from build123d import *

# Parameters (mm, degrees)
SKETCH_1_R             = 28.9
EXTRUDE_1_DEPTH        = 1.6
CHAMFER_1_SIZE         = 0.8
SKETCH_2_R             = 23.75
EXTRUDE_2_DEPTH        = 20
HOLE_WIZARD_M4_1_D     = 3.3
HOLE_WIZARD_M4_1_DEPTH = 9.008579979
HOLE_WIZARD_M4_1_TIP   = 0.991420021
SKETCH_3_R             = 7.5
CUT_EXTRUDE_1_DEPTH    = 4
SKETCH_7_R             = 3.9
EXTRUDE_3_DEPTH        = 3.5
SKETCH_8_R             = 2.34
CUT_EXTRUDE_2_DEPTH    = 10
SKETCH_9_R             = 2
CUT_EXTRUDE_3_DEPTH    = 10


with BuildPart() as part:
    # 草图1 → 凸台-拉伸1 (new body)
    with BuildSketch(Plane(origin=(0, 0, 0), x_dir=(1, 0, 0), z_dir=(0, 1, 0))):
        with Locations(Location((0, 0, 0), (0, 0, 270))):
            Circle(SKETCH_1_R)
    extrude(amount=EXTRUDE_1_DEPTH)

    # 倒角1
    chamfer_1_edges = [part.edges().sort_by_distance(p)[0] for p in [
        (0, 1.6, -28.9),
    ]]
    chamfer(chamfer_1_edges, length=CHAMFER_1_SIZE)

    # 草图2 → 凸台-拉伸2 (add)
    with BuildSketch(Plane.XZ):
        with Locations(Location((0, 0, 0), (0, 0, 270))):
            Circle(SKETCH_2_R)
    extrude(amount=EXTRUDE_2_DEPTH)

    # M4 螺纹孔的螺纹孔钻头1
    with Locations(Plane(origin=(0, 1.6, 0), x_dir=(1, 0, 0), z_dir=(0, 1, 0))):
        with Locations((-17.25, 0), (-8.625, 14.938938215), (8.625, 14.938938215), (17.25, 0), (8.625, -14.938938215), (-8.625, -14.938938215)):
            Hole(HOLE_WIZARD_M4_1_D / 2, depth=HOLE_WIZARD_M4_1_DEPTH)
            with Locations((0, 0, -(HOLE_WIZARD_M4_1_DEPTH + HOLE_WIZARD_M4_1_TIP / 2))):  # 118° drill point
                Cone(0, HOLE_WIZARD_M4_1_D / 2, HOLE_WIZARD_M4_1_TIP, mode=Mode.SUBTRACT)

    # 草图3 → 切除-拉伸1 (cut)
    with BuildSketch(Plane(origin=(0, 1.6, 0), x_dir=(1, 0, 0), z_dir=(0, 1, 0))):
        with Locations(Location((0, 0, 0), (0, 0, 270))):
            Circle(SKETCH_3_R)
        with BuildLine():
            Line((-2.628287969, 9.808904238), (-4.34330439, 16.209432654))
            ThreePointArc((-4.34330439, 16.209432654), (-4.081182154, 17.827981129), (-2.696831759, 18.706605744))
            ThreePointArc((-2.696831759, 18.706605744), (0, 18.9), (2.696831759, 18.706605744))
            ThreePointArc((2.696831759, 18.706605744), (4.081182154, 17.827981129), (4.34330439, 16.209432654))
            Line((4.34330439, 16.209432654), (2.628287969, 9.808904238))
            ThreePointArc((2.628287969, 9.808904238), (1.859855262, 8.699749054), (0.561859251, 8.331075212))
            ThreePointArc((0.561859251, 8.331075212), (0, 8.35), (-0.561859251, 8.331075212))
            ThreePointArc((-0.561859251, 8.331075212), (-1.859855262, 8.699749054), (-2.628287969, 9.808904238))
        make_face()
        with BuildLine():
            Line((9.808904238, 2.628287969), (16.209432654, 4.34330439))
            ThreePointArc((16.209432654, 4.34330439), (17.480075633, 5.379583142), (17.548811672, 7.017778059))
            ThreePointArc((17.548811672, 7.017778059), (16.367880132, 9.45), (14.851979913, 11.688827685))
            ThreePointArc((14.851979913, 11.688827685), (13.398893479, 12.448397987), (11.866128265, 11.866128265))
            Line((11.866128265, 11.866128265), (7.180616269, 7.180616269))
            ThreePointArc((7.180616269, 7.180616269), (6.604276056, 5.960556431), (6.933993149, 4.65212199))
            ThreePointArc((6.933993149, 4.65212199), (7.231312122, 4.175), (7.495852399, 3.678953221))
            ThreePointArc((7.495852399, 3.678953221), (8.464131318, 2.739192623), (9.808904238, 2.628287969))
        make_face()
        with BuildLine():
            Line((7.180616269, -7.180616269), (11.866128265, -11.866128265))
            ThreePointArc((11.866128265, -11.866128265), (13.398893479, -12.448397987), (14.851979913, -11.688827685))
            ThreePointArc((14.851979913, -11.688827685), (16.367880132, -9.45), (17.548811672, -7.017778059))
            ThreePointArc((17.548811672, -7.017778059), (17.480075633, -5.379583142), (16.209432654, -4.34330439))
            Line((16.209432654, -4.34330439), (9.808904238, -2.628287969))
            ThreePointArc((9.808904238, -2.628287969), (8.464131318, -2.739192623), (7.495852399, -3.678953221))
            ThreePointArc((7.495852399, -3.678953221), (7.231312122, -4.175), (6.933993149, -4.65212199))
            ThreePointArc((6.933993149, -4.65212199), (6.604276056, -5.960556431), (7.180616269, -7.180616269))
        make_face()
        with BuildLine():
            Line((-2.628287969, -9.808904238), (-4.34330439, -16.209432654))
            ThreePointArc((-4.34330439, -16.209432654), (-4.081182154, -17.827981129), (-2.696831759, -18.706605744))
            ThreePointArc((-2.696831759, -18.706605744), (0, -18.9), (2.696831759, -18.706605744))
            ThreePointArc((2.696831759, -18.706605744), (4.081182154, -17.827981129), (4.34330439, -16.209432654))
            Line((4.34330439, -16.209432654), (2.628287969, -9.808904238))
            ThreePointArc((2.628287969, -9.808904238), (1.859855262, -8.699749054), (0.561859251, -8.331075212))
            ThreePointArc((0.561859251, -8.331075212), (0, -8.35), (-0.561859251, -8.331075212))
            ThreePointArc((-0.561859251, -8.331075212), (-1.859855262, -8.699749054), (-2.628287969, -9.808904238))
        make_face()
        with BuildLine():
            Line((-9.808904238, -2.628287969), (-16.209432654, -4.34330439))
            ThreePointArc((-16.209432654, -4.34330439), (-17.480075633, -5.379583142), (-17.548811672, -7.017778059))
            ThreePointArc((-17.548811672, -7.017778059), (-16.367880132, -9.45), (-14.851979913, -11.688827685))
            ThreePointArc((-14.851979913, -11.688827685), (-13.398893479, -12.448397987), (-11.866128265, -11.866128265))
            Line((-11.866128265, -11.866128265), (-7.180616269, -7.180616269))
            ThreePointArc((-7.180616269, -7.180616269), (-6.604276056, -5.960556431), (-6.933993149, -4.65212199))
            ThreePointArc((-6.933993149, -4.65212199), (-7.231312122, -4.175), (-7.495852399, -3.678953221))
            ThreePointArc((-7.495852399, -3.678953221), (-8.464131318, -2.739192623), (-9.808904238, -2.628287969))
        make_face()
        with BuildLine():
            Line((-7.180616269, 7.180616269), (-11.866128265, 11.866128265))
            ThreePointArc((-11.866128265, 11.866128265), (-13.398893479, 12.448397987), (-14.851979913, 11.688827685))
            ThreePointArc((-14.851979913, 11.688827685), (-16.367880132, 9.45), (-17.548811672, 7.017778059))
            ThreePointArc((-17.548811672, 7.017778059), (-17.480075633, 5.379583142), (-16.209432654, 4.34330439))
            Line((-16.209432654, 4.34330439), (-9.808904238, 2.628287969))
            ThreePointArc((-9.808904238, 2.628287969), (-8.464131318, 2.739192623), (-7.495852399, 3.678953221))
            ThreePointArc((-7.495852399, 3.678953221), (-7.231312122, 4.175), (-6.933993149, 4.65212199))
            ThreePointArc((-6.933993149, 4.65212199), (-6.604276056, 5.960556431), (-7.180616269, 7.180616269))
        make_face()
    extrude(amount=-CUT_EXTRUDE_1_DEPTH, mode=Mode.SUBTRACT)

    # 草图7 → 凸台-拉伸3 (add)
    with BuildSketch(Plane(origin=(0, -2.4, 0), x_dir=(1, 0, 0), z_dir=(0, 1, 0))):
        with Locations(Location((0, 0, 0), (0, 0, 270))):
            Circle(SKETCH_7_R)
    extrude(amount=EXTRUDE_3_DEPTH)

    # 草图8 → 切除-拉伸2 (cut)
    with BuildSketch(Plane(origin=(0, 1.1, 0), x_dir=(1, 0, 0), z_dir=(0, 1, 0))):
        with Locations(Location((0, 0, 0), (0, 0, 270))):
            Circle(SKETCH_8_R)
    extrude(amount=-CUT_EXTRUDE_2_DEPTH, mode=Mode.SUBTRACT)

    # 草图9 → 切除-拉伸3 (cut)
    with BuildSketch(Plane(origin=(0, -2.4, 0), x_dir=(1, 0, 0), z_dir=(0, 1, 0))):
        with Locations(Location((-12.297560734, 7.1, 0), (0, 0, 270))):
            Circle(SKETCH_9_R)
        with Locations(Location((0, 14.2, 0), (0, 0, 270))):
            Circle(SKETCH_9_R)
        with Locations(Location((12.297560734, 7.1, 0), (0, 0, 270))):
            Circle(SKETCH_9_R)
        with Locations(Location((12.297560734, -7.1, 0), (0, 0, 270))):
            Circle(SKETCH_9_R)
        with Locations(Location((0, -14.2, 0), (0, 0, 270))):
            Circle(SKETCH_9_R)
        with Locations(Location((-12.297560734, -7.1, 0), (0, 0, 270))):
            Circle(SKETCH_9_R)
    extrude(amount=-CUT_EXTRUDE_3_DEPTH, mode=Mode.SUBTRACT)


solid = part.part
Geometry check sheet. Reference: the model listing, model coordinates, mm. Coordinates: 2 decimals unless noted, no trailing zeros. Write each loop counter-clockwise with the first axis right and the second up, starting at its lowest first coordinate (ties: lowest second). Pieces come first, ordered by that corner, then holes. Notation, with made-up numbers: (-28.5, 85.5) -> (-11.5, 85.5) arc R33 cw to (-11.5, 120.5) -> close; hole circle Ø9 at (53, 46.25). An arc over 180 degrees is marked (long way). One line per question, with ' | ' between items.
1. Cross-section at A-A on y = -14.75. Record the cut outline in (x, z).
Answers:
outline: circle Ø47.5 at (0, 0)
2. Draft check along Z on faces 1 (the cylindrical face through (24.369, 0.394, 15.536)), 2 (the cylindrical face through (-8.48, -0.37, -2.73)). Enter one of: +Z half, -Z half, draft (parallel to the pull), parting line (faces both ways), or undercut.
Answers:
face 1: parting line | face 2: undercut
3. Thickness scan on probe 1 along Z at (x, y) = (17.25, -2); probe 2 along Z at (x, y) = (-11.5, -5.25); probe 3 along Z at (x, y) = (-9, -5.25). Record the ranges inside material, lowest first. Write a range as from..to.
Answers:
probe 1: z = -16.32..-7.72, -5.02..-1.65, 1.65..5.02, 7.72..16.32 | probe 2: z = -20.78..-8.93, -5.27..5.27, 8.93..20.78 | probe 3: z = -21.98..-16.55, -13.33..13.33, 16.55..21.98
4. Depth check by flat-ended pin: pin 1 Ø3 at (x, z) = (13.5, -6) entering from +Y; pin 2 Ø1 at (x, z) = (18, -17) entering from -Y; pin 3 Ø8 at (y, z) = (-14.5, 6) entering from -X. Enter the tip coordinate at first touch or a pass-through.
Answers:
pin 1: stops at y = -2.4 | pin 2: stops at y = 0 | pin 3: stops at x = -23.67
